Part model, mm, in its own coordinate system. A direction names the side the tool comes from. Give positions to 0.01 mm unless a question says otherwise; leave off trailing zeros. Order: outer loops, then holes, each group sorted by start corner. A loop starts at its lowest first (then second) coordinate and runs counter-clockwise, first axis right, second up. Notation, with made-up numbers: (37.5, 33.25) - (68.5, 33.25) arc R20 ccw to (68.5, 66.25) - close; hole circle Ø1 at (87.5, 1). An arc over 180 degrees is marked (long way). One line per item, written item: value.
```python
from build123d import *

# Parameters (mm, degrees)
SKETCH1_W           = 8
SKETCH1_H           = 18.5
SKETCH1_R           = 2.25
BOSS_EXTRUDE1_DEPTH = 5.14
BOSS_EXTRUDE2_START = 0.47
SKETCH1_4_W         = 7.2
SKETCH1_4_H         = 7.806654437
BOSS_EXTRUDE2_DEPTH = 4.2


with BuildPart() as part:
    # Sketch1 → Boss-Extrude1 (new body)
    with BuildSketch(Plane(origin=(0, 0, 0), x_dir=(1, 0, 0), z_dir=(0, 1, 0))):
        with Locations((-0.205969798, 1.388672352)):
            Rectangle(SKETCH1_W, SKETCH1_H)
        with Locations((-0.2, -3.25974881)):
            Circle(SKETCH1_R, mode=Mode.SUBTRACT)
        with Locations((-0.2, 6.24025119)):
            Circle(SKETCH1_R, mode=Mode.SUBTRACT)
    extrude(amount=BOSS_EXTRUDE1_DEPTH)

    # Sketch1_4 → Boss-Extrude2 (add)
    with BuildSketch(Plane(origin=(0, 0, 0), x_dir=(1, 0, 0), z_dir=(0, 1, 0)).offset(BOSS_EXTRUDE2_START)):
        with Locations((-0.2, -11.764654867)):
            Rectangle(SKETCH1_4_W, SKETCH1_4_H)
    extrude(amount=BOSS_EXTRUDE2_DEPTH)


solid = part.part
```
1) Slice it at A-A on z = -7.75. Write the cut outline in (x, y), then the cut area to 3 significant figures.
Answer:
outline: (-4.21, 0) - (-1.87, 0) - (-1.87, 5.14) - (-4.21, 5.14) - close; (1.47, 0) - (3.79, 0) - (3.79, 5.14) - (1.47, 5.14) - close
area: 24.0 mm2
2) Wall check: line 1 along Z through (x, y) = (-0.2, 3.85); line 2 along Z through (x, y) = (-1, 1.65); line 3 along Y through (x, z) = (-3, 8.75). Give the ranges that are in metal, low to high. Write a range as [from, to].
Answer:
line 1: z = [-10.64, -8.49], [-3.99, 1.01], [5.51, 15.67]
line 2: z = [-10.64, -8.34], [-4.14, 1.16], [5.36, 15.67]
line 3: y = [0.47, 4.67]
3) Two-plate mould, pull along Z, no slides. Class faces 1 (the face through (0, 3, -10.639)), 2 (the face through (-0.49, 2.53, -8.47)), 3 (the face through (3.4, 3, 12)): pulls with the +Z half, pulls with the -Z half, needs draft (parallel to the pull), parting line crosses it, or undercut.
Answer:
face 1: pulls with the -Z half
face 2: undercut
face 3: needs draft
4) Which spindle directions (+Z, -Z, +X, -X, +Y, -Y) get a long thin tool onto all of the face, cutting with end or side? Do faces 4 (the face through (-3.8, 3, 12)), 5 (the face through (0, 4.67, 12)), 6 (the face through (0, 0.47, 12)). Say none if no direction does.
Answer:
face 4: +Z, -X, +Y, -Y
face 5: +Z, +X, -X, +Y
face 6: +Z, +X, -X, -Y
5) Slice it at C-C on y = 4.25. Write the cut outline in (x, z), then the cut area to 3 significant figures.
Answer:
outline: (-4.21, -10.64) - (3.79, -10.64) - (3.79, 7.86) - (3.4, 7.86) - (3.4, 15.67) - (-3.8, 15.67) - (-3.8, 7.86) - (-4.21, 7.86) - close; hole circle Ø4.5 at (-0.2, -6.24); hole circle Ø4.5 at (-0.2, 3.26)
area: 172 mm2
6) Slice it at B-B on x = 3. Write the cut outline in (y, z), then the cut area to 3 significant figures.
Answer:
outline: (0, -10.64) - (5.14, -10.64) - (5.14, 7.86) - (4.67, 7.86) - (4.67, 15.67) - (0.47, 15.67) - (0.47, 7.86) - (0, 7.86) - close
area: 128 mm2
7) Slice it at D-D on x = -0.2. Write the cut outline in (y, z), then the cut area to 3 significant figures.
Answer:
outline: (0, -10.64) - (5.14, -10.64) - (5.14, -8.49) - (0, -8.49) - close; (0, -3.99) - (5.14, -3.99) - (5.14, 1.01) - (0, 1.01) - close; (0, 5.51) - (5.14, 5.51) - (5.14, 7.86) - (4.67, 7.86) - (4.67, 15.67) - (0.47, 15.67) - (0.47, 7.86) - (0, 7.86) - close
area: 81.6 mm2
8) Drop flat-ended pins along their axis: P1, Ø1.3, axis at y = 2.5, z = 13.5, coming from the +X side; P2, Ø3.5, axis at x = -1, z = 12.5, coming from the -Y side; P3, Ø1.3, axis at y = 2, z = 10.5, coming from the -X side. Give the stop position or say it passes through.
Answer:
P1: stops at x = 3.4
P2: stops at y = 0.47
P3: stops at x = -3.8
